```python
from build123d import *

# Parameters (mm, degrees)
SKETCH1_W                        = 60
SKETCH1_H                        = 16
BOSS_EXTRUDE1_DEPTH              = 10
SKETCH3_W                        = 20.254
SKETCH3_H                        = 13.746
CUT_EXTRUDE1_DEPTH               = 8
M2_5_CLEARANCE_HOLE1_D           = 3.1
M2_5_CLEARANCE_HOLE1_CSINK_D     = 3.15
M2_5_CLEARANCE_HOLE1_CSINK_ANGLE = 90
BOSS_EXTRUDE4_DEPTH              = 35
CUT_EXTRUDE8_DEPTH               = 107.825342634
CUT_EXTRUDE8_DEPTH_BACK          = 107.825342634
SKETCH14_OUTSIDE_W               = 163.346
SKETCH14_OUTSIDE_H               = 64.796
FILLET6_R                        = 3


with BuildPart() as part:
    # Sketch1 → Boss-Extrude1 (new body)
    with BuildSketch(Plane(origin=(0, 0, 0), x_dir=(1, 0, 0), z_dir=(0, 1, 0))):
        Rectangle(SKETCH1_W, SKETCH1_H)
    extrude(amount=BOSS_EXTRUDE1_DEPTH)

    # Sketch3 → Cut-Extrude1 (cut)
    with BuildSketch(Plane(origin=(0, 0, 0), x_dir=(1, 0, 0), z_dir=(0, 1, 0))):
        with Locations((19.873, 0)):
            Rectangle(SKETCH3_W, SKETCH3_H)
    extrude(amount=CUT_EXTRUDE1_DEPTH, mode=Mode.SUBTRACT)

    # M2.5 Clearance Hole1 (through all)
    with Locations(Plane.XY.offset(8)):
        with Locations((15.2, 4), (25.2, 4)):
            CounterSinkHole(M2_5_CLEARANCE_HOLE1_D / 2, M2_5_CLEARANCE_HOLE1_CSINK_D / 2, counter_sink_angle=M2_5_CLEARANCE_HOLE1_CSINK_ANGLE)

    # Sketch12 → Boss-Extrude4 (add)
    with BuildSketch(Plane(origin=(0, 10, 0), x_dir=(1, 0, 0), z_dir=(0, 1, 0))):
        Polygon((-30, 8), (-103.550247845, 7.999936172), (-103.550247845, -3.1914e-05), (-103.550247845, -8), (-30, -8), align=None)
    extrude(amount=-BOSS_EXTRUDE4_DEPTH)

    # Sketch14 outside → Cut-Extrude8 (cut, two sides: drawn at the far end of the back side and taken through both)
    with BuildSketch(Plane.XY.offset(-CUT_EXTRUDE8_DEPTH_BACK)):
        with Locations((-36.775, -7.5)):
            Rectangle(SKETCH14_OUTSIDE_W, SKETCH14_OUTSIDE_H)
        with BuildLine():
            Line((30, 0), (-30, 0))
            ThreePointArc((-30, 0), (-44.809706125, -4.518239103), (-54.575111815, -16.534009232))
            Line((-54.575111815, -16.534009232), (-65.929573082, -19.931975488))
            ThreePointArc((-65.929573082, -19.931975488), (-53.381923459, 1.536604003), (-30, 10))
            Line((-30, 10), (30, 10))
            Line((30, 10), (30, 0))
        make_face(mode=Mode.SUBTRACT)
    extrude(amount=CUT_EXTRUDE8_DEPTH + CUT_EXTRUDE8_DEPTH_BACK, mode=Mode.SUBTRACT)

    # Fillet6
    fillet6_edges = [part.edges().sort_by_distance(p)[0] for p in [
        (-54.575111815, -16.534009232, 1.0663e-05),
        (-60.252342448, -18.23299236, -7.999973747),
        (-65.929573082, -19.931975488, 1.559e-05),
        (-60.252342448, -18.23299236, 8),
    ]]
    fillet(fillet6_edges, radius=FILLET6_R)


solid = part.part
```
Model file for the job. Use its own axes, mm. A direction names the side the tool comes from. Coordinates: 2 decimals unless noted, no trailing zeros. Write each loop counter-clockwise with the first axis right and the second up, starting at its lowest first coordinate (ties: lowest second). Pieces come first, ordered by that corner, then holes. Notation, with made-up numbers: (89.25, 28.5) - (146.25, 28.5) arc R29 ccw to (146.25, 67.5) - close; hole circle Ø11 at (-30, 0.5). An arc over 180 degrees is marked (long way). Use a Markdown table: item, result. Add a question column.
Item 1: Band-saw the part on A-A, the plane x = 15.2. Write the cut outline in (y, z) (3 decimals).
Item 2: Band-saw the part on D-D, the plane x = -19. Write the cut outline in (y, z), and give its area (3 significant figures).
Item 3: Drill centre lines: line 1 along Z through (x, y) = (25, 6.75); line 2 along X through (y, z) = (4, 7.4); line 3 along Y through (x, z) = (25.2, 7.35). Where is each one in solid material? Low to high.
Item 4: Two-plate mould, pull along Z, no slides. Class faces 3 (the face through (30, 8.3, 0.1)), 4 (the face through (20, 8, 0)), 5 (the face through (-18, 3, 8)): pulls with the +Z half, pulls with the -Z half, needs draft (parallel to the pull), parting line crosses it, or undercut.
Item 5: Band-saw the part on C-C, the plane z = 2.25. Write the cut outline in (x, y).
Item 6: Drop flat-ended pins along their axis: pin 1 (3.5 mm diameter, centred on x = 25.2, y = 4, fed in from +Z); pin 2 (5 mm diameter, centred on x = -34.5, z = 1, fed in from +Y); pin 3 (8 mm diameter, centred on x = 8.5, z = -3.5, fed in from -Y); pin 4 (2 mm diameter, centred on y = -5, z = -5.5, fed in from +X). Give the stop position or say it passes through.
Item 7: Band-saw the part on B-B, the plane y = 4. Give the number of separate pieces and of enclosed holes in the cut face, and give its area (3 significant figures).
Item 8: 3-axis set-ups, long thin cutter, end or side, ignore diameter. For faces 1 (the face through (9.746, 4, 0)), 2 (the face through (-58.237, -16.266, -7.476)): which of +Z, -Z, +X, -X, +Y, -Y reach the whole face in a straight line?
A:
| question | item | result |
|---|---|---|
| 1 | outline | (0, -8) - (2.45, -8) - (2.45, -6.873) - (0, -6.873) - close; (0, 6.873) - (2.45, 6.873) - (2.45, 7.975) - (2.425, 8) - (0, 8) - close; (5.55, -8) - (10, -8) - (10, 8) - (5.575, 8) - (5.55, 7.975) - (5.55, 6.873) - (8, 6.873) - (8, -6.873) - (5.55, -6.873) - close |
| 2 | outline | (0, -8) - (10, -8) - (10, 8) - (0, 8) - close |
| 2 | area | 160 mm² |
| 3 | line 1 | z = -8 to -6.87, 6.87 to 8 |
| 3 | line 2 | x = -50.06 to 13.65, 16.75 to 23.65, 26.75 to 30 |
| 3 | line 3 | y = 0 to 2.45, 5.55 to 10 |
| 4 | face 3 | needs draft |
| 4 | face 4 | undercut |
| 4 | face 5 | pulls with the +Z half |
| 5 | outline | (-64.51, -14.54) arc R3 ccw to (-60.81, -18.4) - (-55.91, -16.93) arc R3 ccw to (-54.05, -15.33) arc R26.53 cw to (-30, 0) - (9.75, 0) - (9.75, 8) - (30, 8) - (30, 10) - (-30, 10) arc R36.53 ccw to start |
| 6 | pin 1 | stops at z = 8 |
| 6 | pin 2 | stops at y = 9.95 |
| 6 | pin 3 | stops at y = 0 |
| 6 | pin 4 | stops at x = -44.01 |
| 7 | separate pieces | 5 |
| 7 | enclosed holes | 0 |
| 7 | area | 989 mm² |
| 8 | face 1 | +X, -Y |
| 8 | face 2 | -Z, +X, -Y |
